from build123d import *

# Parameters (mm, degrees)
SKETCH1_W               = 100
SKETCH1_H               = 50
BOSS_EXTRUDE1_DEPTH     = 30
SKETCH2_R               = 2.5
CUT_EXTRUDE1_DEPTH      = 108.354552768
FILLET1_R               = 5
CUT_EXTRUDE2_REACH      = 65.443
CUT_EXTRUDE2_END_RADIUS = 2.5
SKETCH3_R               = 2.5


with BuildPart() as part:
    # Sketch1 → Boss-Extrude1 (new body)
    with BuildSketch(Plane.XY):
        Rectangle(SKETCH1_W, SKETCH1_H)
    extrude(amount=BOSS_EXTRUDE1_DEPTH)

    # Sketch2 → Cut-Extrude1 (cut, through all)
    with BuildSketch(Plane(origin=(50, 0, 0), x_dir=(0, 0, -1), z_dir=(1, 0, 0))):
        with Locations(Location((-10, 15, 0), (0, 0, 90))):
            Circle(SKETCH2_R)
        with Locations(Location((-10, -15, 0), (0, 0, 90))):
            Circle(SKETCH2_R)
    extrude(amount=-CUT_EXTRUDE1_DEPTH, mode=Mode.SUBTRACT)

    # Fillet1
    fillet1_edges = [part.edges().sort_by_distance(p)[0] for p in [
        (0, -25, 0),
        (-50, 0, 0),
        (0, 25, 0),
        (50, 0, 0),
    ]]
    fillet(fillet1_edges, radius=FILLET1_R)

    # Cut-Extrude2: up to this cylinder (the profile starts outside it)
    cut_extrude2_end = Plane(origin=(0, 15, 10), z_dir=(1, 0, 0)) * Cylinder(CUT_EXTRUDE2_END_RADIUS, 196.886, mode=Mode.PRIVATE)
    # Sketch3 → Cut-Extrude2 (cut, up to the surface)
    with BuildSketch(Plane(origin=(0, 0, 0), x_dir=(-1, 0, 0), z_dir=(0, 0, -1)), mode=Mode.PRIVATE) as cut_extrude2_sk1:
        with Locations((-30, 15)):
            Circle(SKETCH3_R)
    cut_extrude2_tool1 = extrude(cut_extrude2_sk1.sketch, amount=-CUT_EXTRUDE2_REACH, mode=Mode.PRIVATE) - cut_extrude2_end
    add(cut_extrude2_tool1.solids().sort_by_distance((30, 15, 0))[0], mode=Mode.SUBTRACT)
    # Sketch3 → Cut-Extrude2 (cut, up to the surface)
    with BuildSketch(Plane(origin=(0, 0, 0), x_dir=(-1, 0, 0), z_dir=(0, 0, -1)), mode=Mode.PRIVATE) as cut_extrude2_sk2:
        with Locations((30, 15)):
            Circle(SKETCH3_R)
    cut_extrude2_tool2 = extrude(cut_extrude2_sk2.sketch, amount=-CUT_EXTRUDE2_REACH, mode=Mode.PRIVATE) - cut_extrude2_end
    add(cut_extrude2_tool2.solids().sort_by_distance((-30, 15, 0))[0], mode=Mode.SUBTRACT)
    # Sketch3 → Cut-Extrude2 (cut, up to the surface)
    with BuildSketch(Plane(origin=(0, 0, 0), x_dir=(-1, 0, 0), z_dir=(0, 0, -1)), mode=Mode.PRIVATE) as cut_extrude2_sk3:
        with Locations((0, 15)):
            Circle(SKETCH3_R)
    cut_extrude2_tool3 = extrude(cut_extrude2_sk3.sketch, amount=-CUT_EXTRUDE2_REACH, mode=Mode.PRIVATE) - cut_extrude2_end
    add(cut_extrude2_tool3.solids().sort_by_distance((0, 15, 0))[0], mode=Mode.SUBTRACT)


solid = part.part
Geometry check sheet. Reference: the model listing, model coordinates, mm. A direction names the side the tool comes from. Give positions to 0.01 mm unless a question says otherwise; leave off trailing zeros. Order: outer loops, then holes, each group sorted by start corner. A loop starts at its lowest first (then second) coordinate and runs counter-clockwise, first axis right, second up. Notation, with made-up numbers: (89.5, 69.5) - (140.5, 69.5) arc R27 cw to (140.5, 90.5) - close; hole circle Ø9 at (64.25, 87). An arc over 180 degrees is marked (long way). Use one line per item in the form item = value.
1) Sectioned sample at A-A (y = 15). Record the boundary of the cut face in (x, z), and give its area (3 significant figures).
Working result:
outline = (-50, 5) arc R5 ccw to (-45, 0) - (-32.5, 0) - (-32.5, 7.5) - (-50, 7.5) - close; (-50, 12.5) - (50, 12.5) - (50, 30) - (-50, 30) - close; (-27.5, 0) - (-2.5, 0) - (-2.5, 7.5) - (-27.5, 7.5) - close; (2.5, 0) - (27.5, 0) - (27.5, 7.5) - (2.5, 7.5) - close; (32.5, 0) - (45, 0) arc R5 ccw to (50, 5) - (50, 7.5) - (32.5, 7.5) - close
area = 2,380 mm^2
2) Sectioned sample at B-B (x = 14). Record the boundary of the cut face in (y, z).
Working result:
outline = (-25, 5) arc R5 ccw to (-20, 0) - (20, 0) arc R5 ccw to (25, 5) - (25, 30) - (-25, 30) - close; hole circle Ø5 at (-15, 10); hole circle Ø5 at (15, 10)
3) Sectioned sample at C-C (y = -15). Record the boundary of the cut face in (x, z).
Working result:
outline = (-50, 5) arc R5 ccw to (-45, 0) - (45, 0) arc R5 ccw to (50, 5) - (50, 7.5) - (-50, 7.5) - close; (-50, 12.5) - (50, 12.5) - (50, 30) - (-50, 30) - close
4) Sectioned sample at D-D (x = 30). Record the boundary of the cut face in (y, z), and give its area (3 significant figures).
Working result:
outline = (-25, 5) arc R5 ccw to (-20, 0) - (12.5, 0) - (12.5, 10) arc R2.5 cw to (17.5, 10) - (17.5, 0) - (20, 0) arc R5 ccw to (25, 5) - (25, 30) - (-25, 30) - close; hole circle Ø5 at (-15, 10)
area = 1,410 mm^2
5) Access from +Z, -Z, +X, -X, +Y, -Y to the whole of each face (thin tool, end or side, straight path). Record for faces 4 (the face through (-1, 25, 17)), 5 (the face through (-2.31, 14.04, 3.82)).
Working result:
face_4 = +Z, -Z, +X, -X, +Y
face_5 = -Z
6) Draft check along Z on faces 1 (the face through (-1, 0, 30)), 2 (the face through (27.69, 14.04, 3.82)), 3 (the face through (0.7, 14.67, 12.48)). Enter one of: released by +Z, released by -Z, zero draft, split by the parting line, or undercut.
Working result:
face_1 = released by +Z
face_2 = zero draft
face_3 = undercut
7) Depth check by flat-ended pin: pin 1 Ø2 at (x, z) = (22.5, 3) entering from +Y; pin 2 Ø4 at (x, y) = (30, 15) entering from -Z. Enter the tip coordinate at first touch or a pass-through.
Working result:
pin_1 = 24.9
pin_2 = 11.5
8) Material ranges on probe 1 along Z at (x, y) = (-22, -15); probe 2 along Y at (x, z) = (30, 5.5); probe 3 along Y at (x, z) = (27, 10.5), recorded low to high. Write a range as from..to.
Working result:
probe_1 = 0..7.5, 12.5..30
probe_2 = -25..12.5, 17.5..25
probe_3 = -25..-17.45, -12.55..12.55, 17.45..25
